Source: CAD feature listing. Evaluate the final solid. Frame: model axes, mm. Face numbers are marked on the shaded views. Round coordinates to 2 decimals unless told otherwise and drop trailing zeros. Order: outer loops, then holes, each group sorted by start corner. A loop starts at its lowest first (then second) coordinate and runs counter-clockwise, first axis right, second up. Notation, with made-up numbers: (74.25, 48.5) -> (94.25, 48.5) arc R23 cw to (94.25, 70.5) -> close; hole circle Ø4 at (39, 29). An arc over 180 degrees is marked (long way). Use a Markdown table: item, result. Add a question column.
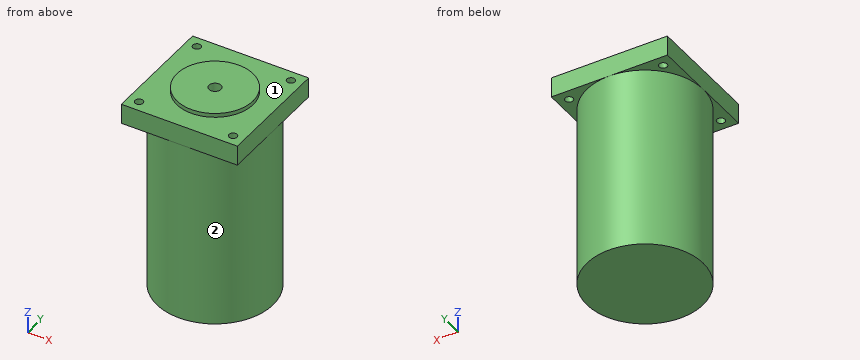
```python
from build123d import *

# Parameters (mm, degrees)
SKETCH1_R           = 19
BOSS_EXTRUDE1_DEPTH = 2
SKETCH3_W           = 58
SKETCH3_H           = 58
BOSS_EXTRUDE2_DEPTH = 10
SKETCH4_R           = 29
BOSS_EXTRUDE3_DEPTH = 91.5
SKETCH5_R           = 2
CUT_EXTRUDE1_DEPTH  = 10
SKETCH6_R           = 3
CUT_EXTRUDE2_DEPTH  = 12


with BuildPart() as part:
    # Sketch1 → Boss-Extrude1 (new body)
    with BuildSketch(Plane.XY):
        Circle(SKETCH1_R)
    extrude(amount=-BOSS_EXTRUDE1_DEPTH)

    # Sketch3 → Boss-Extrude2 (add)
    with BuildSketch(Plane(origin=(0, 0, -2), x_dir=(-1, 0, 0), z_dir=(0, 0, -1))):
        Rectangle(SKETCH3_W, SKETCH3_H)
    extrude(amount=BOSS_EXTRUDE2_DEPTH)

    # Sketch4 → Boss-Extrude3 (add)
    with BuildSketch(Plane(origin=(0, 0, -12), x_dir=(-1, 0, 0), z_dir=(0, 0, -1))):
        Circle(SKETCH4_R)
    extrude(amount=BOSS_EXTRUDE3_DEPTH)

    # Sketch5 → Cut-Extrude1 (cut)
    with BuildSketch(Plane.XY.offset(-2)):
        with Locations((-23.5, 23.5)):
            Circle(SKETCH5_R)
        with Locations((23.5, 23.5)):
            Circle(SKETCH5_R)
        with Locations((23.5, -23.5)):
            Circle(SKETCH5_R)
        with Locations((-23.5, -23.5)):
            Circle(SKETCH5_R)
    extrude(amount=-CUT_EXTRUDE1_DEPTH, mode=Mode.SUBTRACT)

    # Sketch6 → Cut-Extrude2 (cut)
    with BuildSketch(Plane.XY):
        Circle(SKETCH6_R)
    extrude(amount=-CUT_EXTRUDE2_DEPTH, mode=Mode.SUBTRACT)


solid = part.part
```
1) Line query: probe 1 along Y at (x, z) = (23.5, -8.25); probe 2 along Y at (x, z) = (0, -4); probe 3 along Z at (x, y) = (-8, -24). Output: solid intervals per line, ascending. Write a range as from..to.
2) Draft query along X for the marked faces 1 and 2. Return one class per face: pulls with the +X half, pulls with the -X half, needs draft (parallel to the pull), parting line crosses it, or undercut.
3) Section A-A on x = 23.5. Output: boundary loops of the cut face in (y, z).
4) Section C-C on y = -7.5. Output: boundary loops of the cut face in (x, z).
5) First-contact query: pin 1 Ø2.5 at (x, y) = (-23.5, -23.5) entering from +Z; pin 2 Ø5 at (x, y) = (-19, -19) entering from +Z; pin 3 Ø3 at (x, z) = (19, -76.5) entering from -Y; pin 4 Ø1.5 at (y, z) = (8.5, -15.5) entering from +X. Flat tips, straight axial feed; report the tip coordinate or a pass-through.
6) Section D-D on z = -64. Output: boundary loops of the cut face in (x, y).
Conclusion:
| question | item | result |
|---|---|---|
| 1 | probe 1 | y = -29..-25.5, -21.5..21.5, 25.5..29 |
| 1 | probe 2 | y = -29..-3, 3..29 |
| 1 | probe 3 | z = -103.5..-2 |
| 2 | face 1 | needs draft |
| 2 | face 2 | parting line crosses it |
| 3 | outline | (-29, -12) -> (-25.5, -12) -> (-25.5, -2) -> (-29, -2) -> close; (-21.5, -12) -> (-16.99, -12) -> (-16.99, -103.5) -> (16.99, -103.5) -> (16.99, -12) -> (21.5, -12) -> (21.5, -2) -> (-21.5, -2) -> close; (25.5, -12) -> (29, -12) -> (29, -2) -> (25.5, -2) -> close |
| 4 | outline | (-29, -12) -> (-28.01, -12) -> (-28.01, -103.5) -> (28.01, -103.5) -> (28.01, -12) -> (29, -12) -> (29, -2) -> (17.46, -2) -> (17.46, 0) -> (-17.46, 0) -> (-17.46, -2) -> (-29, -2) -> close |
| 5 | pin 1 | passes through |
| 5 | pin 2 | stops at z = -2 |
| 5 | pin 3 | stops at y = -23.12 |
| 5 | pin 4 | stops at x = 27.95 |
| 6 | outline | circle Ø58 at (0, 0) |
